from build123d import *

# Parameters (mm, degrees)
RESSALTO_EXTRUS_O1_DEPTH = 55.1
ESBO_O5_W                = 9.4
ESBO_O5_H                = 2
RESSALTO_EXTRUS_O2_DEPTH = 3.05
ESBO_O8_W                = 3.5
ESBO_O8_H                = 3.5
CORTE_EXTRUS_O6_DEPTH    = 3.5
ESBO_O9_W                = 10
ESBO_O9_H                = 20
CORTE_EXTRUS_O7_DEPTH    = 71.482001249
FILETE1_R                = 1


with BuildPart() as part:
    # Esboço1 → Ressalto-extrusão1 (new body)
    with BuildSketch(Plane.XY):
        with BuildLine():
            Line((0, 0), (40.7, 0))
            Line((40.7, 0), (40.7, 4.2))
            Line((40.7, 4.2), (34.5, 4.2))
            Line((34.5, 4.2), (34.5, 1.6))
            Line((34.5, 1.6), (3.614566097, 1.6))
            ThreePointArc((3.614566097, 1.6), (2.284269322, 2.106577592), (1.627871083, 3.369689511))
            Line((1.627871083, 3.369689511), (1.531616141, 4.2))
            Line((1.531616141, 4.2), (-3.796013859, 4.2))
            Line((-3.796013859, 4.2), (-3.796013859, 0))
            Line((-3.796013859, 0), (0, 0))
        make_face()
    extrude(amount=RESSALTO_EXTRUS_O1_DEPTH)

    # Esboço5 → Ressalto-extrusão2 (add)
    with BuildSketch(Plane(origin=(40.7, 0, 0), x_dir=(0, 0, -1), z_dir=(1, 0, 0))):
        with Locations((-13.6, 1.7)):
            Rectangle(ESBO_O5_W, ESBO_O5_H)
        with Locations((-41.5, 1.7)):
            Rectangle(ESBO_O5_W, ESBO_O5_H)
    extrude(amount=RESSALTO_EXTRUS_O2_DEPTH)

    # Esboço8 → Corte-extrusão6 (cut)
    with BuildSketch(Plane(origin=(0, 4.2, 0), x_dir=(1, 0, 0), z_dir=(0, 1, 0))):
        with Locations((-1.132198859, -51.35)):
            Rectangle(ESBO_O8_W, ESBO_O8_H)
        with Locations((-1.132198859, -3.75)):
            Rectangle(ESBO_O8_W, ESBO_O8_H)
    extrude(amount=-CORTE_EXTRUS_O6_DEPTH, mode=Mode.SUBTRACT)

    # Esboço9 → Corte-extrusão7 (cut, through all)
    with BuildSketch(Plane.XZ):
        with Locations((1.203986141, 27.55)):
            Rectangle(ESBO_O9_W, ESBO_O9_H)
    extrude(amount=-CORTE_EXTRUS_O7_DEPTH, mode=Mode.SUBTRACT)

    # Filete1
    filete1_edges = [part.edges().sort_by_distance(p)[0] for p in [
        (6.203986141, 0.8, 37.55),
        (6.203986141, 0.8, 17.55),
    ]]
    fillet(filete1_edges, radius=FILETE1_R)


solid = part.part
Geometry: final body of the model. Coordinates: model frame, mm. A direction names the side the tool comes from. Give positions to 0.01 mm unless a question says otherwise; leave off trailing zeros. Loops run counter-clockwise (first coordinate to the right, second up) from the corner with the lowest first, then second, coordinate; pieces in that order, holes last. Notation, with made-up numbers: M 3.5,-2.75 L 8.5,-2.75 A28 cw 8.5,33.25 Z; hole C 12,16 d4. An arc over 180 degrees is marked long. Put each result on its own line as item: value. Start each with the question number.
1) Cut plane A-A (z = 16). Output: boundary loops of the cut face in (x, y), then the cut area to 3 significant figures.
2) Cut plane D-D (z = 8). Output: boundary loops of the cut face in (x, y).
3) Access query for faces 1 (the cylindrical face through (2.3, 2.093, 8.652)), 2 (the flat face through (-2.882, 2, 51)), 3 (the flat face through (42, 2, 36.8)), 4 (the flat face through (18, 1, 0)), 5 (the flat face through (0, 2, 37.55)). Directions: +Z, -Z, +X, -X, +Y, -Y. A direction counts if a zero-diameter tool reaches every point of the face in a straight line with its end or side. Return the directions, or none.
4) Pull-direction query (X, two-part tool) for faces 6 (the flat face through (-1, 2, 2)), 7 (the flat face through (38, 4.2, 27)), 8 (the flat face through (6.204, 1, 27)); classes: pulls with the +X half, pulls with the -X half, needs draft (parallel to the pull), parting line crosses it, or undercut.
5) Ray query, line 1 along X through (y, z) = (3.55, 51.5); line 2 along Y through (x, z) = (12, 5); line 3 along X through (y, z) = (0.25, 38). Return the intervals inside material, ascending.
6) Contact query for flat-ended pins moving along their axis: pin 1 (1.6 mm diameter, centred on x = 42.5, y = 2, fed in from -Z); pin 2 (1.8 mm diameter, centred on y = 3, z = 4, fed in from +X); pin 3 (0.9 mm diameter, centred on x = 42.5, z = 43, fed in from -Y). Output: stop coordinate, or through.
7) Cut plane B-B (x = 2.5). Output: boundary loops of the cut face in (y, z).
8) Cut plane C-C (x = 8.5). Output: boundary loops of the cut face in (y, z).
Verdict:
1. outline: M -3.8,0 L 40.7,0 L 40.7,0.7 L 43.75,0.7 L 43.75,2.7 L 40.7,2.7 L 40.7,4.2 L 34.5,4.2 L 34.5,1.6 L 3.61,1.6 A2 cw 1.63,3.37 L 1.53,4.2 L -3.8,4.2 Z
1. area: 108 mm2
2. outline: M -3.8,0 L 40.7,0 L 40.7,4.2 L 34.5,4.2 L 34.5,1.6 L 3.61,1.6 A2 cw 1.63,3.37 L 1.53,4.2 L -3.8,4.2 Z
3. face 1: +Z, -Z, +Y
3. face 2: +Y
3. face 3: +X, +Y, -Y
3. face 4: -Z, +X, -X, +Y, -Y
3. face 5: -X, +Y, -Y
4. face 6: undercut
4. face 7: needs draft
4. face 8: pulls with the -X half
5. line 1: -3.8 to -2.88, 0.62 to 1.61, 34.5 to 40.7
5. line 2: 0 to 1.6
5. line 3: -3.8 to 40.7
6. pin 1: z = 8.9
6. pin 2: x = 40.7
6. pin 3: y = 0.7
7. outline: M 0,0 L 1.94,0 L 1.94,17.55 L 0,17.55 Z; M 0,37.55 L 1.94,37.55 L 1.94,55.1 L 0,55.1 Z
8. outline: M 0,0 L 1.6,0 L 1.6,55.1 L 0,55.1 Z
